from build123d import *

# Parameters (mm, degrees)
BOSS_EXTRUDE1_DEPTH       = 279.4
SKETCH2_R                 = 3.175
CUT_EXTRUDE1_DEPTH        = 51.8
F_4_40_TAPPED_HOLE1_D     = 2.2606
F_4_40_TAPPED_HOLE1_DEPTH = 3.175


with BuildPart() as part:
    # Sketch1 → Boss-Extrude1 (new body)
    with BuildSketch(Plane(origin=(0, 0, 0), x_dir=(1, 0, 0), z_dir=(0, 1, 0))):
        Polygon((-25.4, 25.4), (-25.4, 0), (25.4, 0), (25.4, 25.4), (22.225, 25.4), (22.225, 3.175), (-22.225, 3.175), (-22.225, 25.4), align=None)
    extrude(amount=BOSS_EXTRUDE1_DEPTH)

    # Sketch2 → Cut-Extrude1 (cut, through all)
    with BuildSketch(Plane(origin=(25.4, 0, 0), x_dir=(0, 0, -1), z_dir=(1, 0, 0))):
        with Locations((15.875, 266.7)):
            Circle(SKETCH2_R)
    extrude(amount=-CUT_EXTRUDE1_DEPTH, mode=Mode.SUBTRACT)

    # #4-40 Tapped Hole1
    with Locations(Plane.XY):
        with Locations((0, 146.05), (0, 6.35)):
            Hole(F_4_40_TAPPED_HOLE1_D / 2, depth=F_4_40_TAPPED_HOLE1_DEPTH)


solid = part.part
The model under review builds one solid part; all positions refer to its coordinate system, in mm. A direction names the side the tool comes from. Coordinates: 2 decimals unless noted, no trailing zeros. Write each loop counter-clockwise with the first axis right and the second up, starting at its lowest first coordinate (ties: lowest second). Pieces come first, ordered by that corner, then holes. Notation, with made-up numbers: (46, 75.25) - (82, 75.25) arc R6 cw to (82, 79.25) - close; hole circle Ø11 at (59.25, 31.5). An arc over 180 degrees is marked (long way). Answer as a JSON object with one key per item and string values. Group by question number.
1. Clearance check with flat-ended pins moving along their axes: pin 1 Ø8.5 at (y, z) = (266.7, -15.875) entering from -X; pin 2 Ø1 at (x, y) = (19.5, 152.5) entering from -Z (3 decimals); pin 3 Ø1.4 at (x, y) = (0, 6.35) entering from +Z. State where each tip first meets the part, or that it passes through.
2. To check wall thickness, follow probe 1 along Y at (x, z) = (0, -1.2); probe 2 along X at (y, z) = (238, -7.5) (3 decimals); probe 3 along Z at (x, y) = (-12, 167) (3 decimals). State the ranges of each line that lie inside material, in increasing order.
3. Machinability: for faces 5 (the face through (-22.225, 138, -14)), 6 (the face through (25.4, 138, -13)), which of the approach directions +Z, -Z, +X, -X, +Y, -Y give a long, thin tool a straight path to every point of the face, cutting with its end or side? Answer none if there is none.
4. Add section A-A (y = 266.7). Give the boundary of the cut face in (x, z) (3 decimals).
5. Mouldability with a two-part tool opening along Y and no side actions: class faces 1 (the face through (23.835, 269.848, -15.462)), 2 (the face through (0, 138, -3.175)), 3 (the face through (2, 0, -2)), 4 (the face through (-23.79, 269.848, -15.462)) as pulls with the +Y half, pulls with the -Y half, needs draft (parallel to the pull), parting line crosses it, or undercut.
6. Add section B-B (y = 80). Give the boundary of the cut face in (x, z) (3 decimals).
7. Add section D-D (x = 16.5). Give the boundary of the cut face in (y, z) (3 decimals).
8. Add section C-C (z = -15.5). Give the boundary of the cut face in (x, y) (3 decimals).
Findings:
{
 "1": {"pin 1": "x = -25.4", "pin 2": "z = -3.175", "pin 3": "through"},
 "2": {"probe 1": "0 to 5.22, 7.48 to 144.92, 147.18 to 279.4", "probe 2": "-25.4 to -22.225, 22.225 to 25.4", "probe 3": "-3.175 to 0"},
 "3": {"face 5": "-Z, +Y, -Y", "face 6": "+Z, -Z, +X, +Y, -Y"},
 "4": {"outline": "(-25.4, -25.4) - (-22.225, -25.4) - (-22.225, -19.05) - (-25.4, -19.05) - close; (-25.4, -12.7) - (-22.225, -12.7) - (-22.225, -3.175) - (22.225, -3.175) - (22.225, -12.7) - (25.4, -12.7) - (25.4, 0) - (-25.4, 0) - close; (22.225, -25.4) - (25.4, -25.4) - (25.4, -19.05) - (22.225, -19.05) - close"},
 "5": {"face 1": "undercut", "face 2": "needs draft", "face 3": "pulls with the -Y half", "face 4": "undercut"},
 "6": {"outline": "(-25.4, -25.4) - (-22.225, -25.4) - (-22.225, -3.175) - (22.225, -3.175) - (22.225, -25.4) - (25.4, -25.4) - (25.4, 0) - (-25.4, 0) - close"},
 "7": {"outline": "(0, -3.175) - (279.4, -3.175) - (279.4, 0) - (0, 0) - close"},
 "8": {"outline": "(-25.4, 0) - (-22.225, 0) - (-22.225, 263.547) - (-25.4, 263.547) - close; (-25.4, 269.853) - (-22.225, 269.853) - (-22.225, 279.4) - (-25.4, 279.4) - close; (22.225, 0) - (25.4, 0) - (25.4, 263.547) - (22.225, 263.547) - close; (22.225, 269.853) - (25.4, 269.853) - (25.4, 279.4) - (22.225, 279.4) - close"}
}
